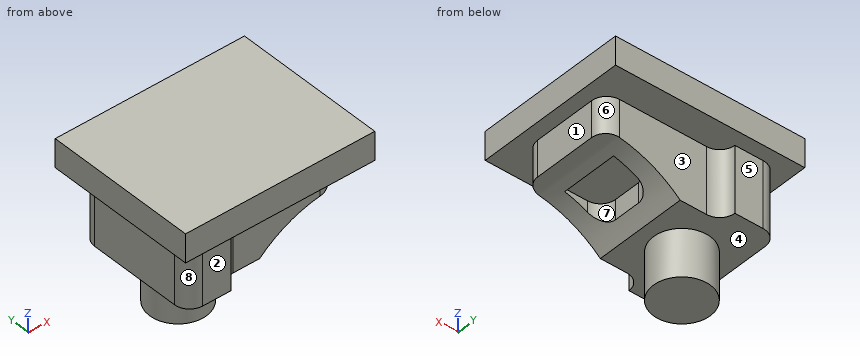
Autodesk Inventor part; units mm, degrees
ref_plane "YZ Plane" through (0, 0, 0) normal (1, 0, 0) x (0, 1, 0)
ref_plane "XZ Plane" through (0, 0, 0) normal (0, 1, 0) x (-1, 0, 0)
ref_plane "XY Plane" through (0, 0, 0) normal (0, 0, 1) x (1, 0, 0)
sketch "Sketch1" plane through (0, 0, 0) normal (0, 0, 1) x (1, 0, 0)
  line L0 (-50, 40) -> (50, 40)
  line L1 (50, 40) -> (50, -40)
  line L2 (50, -40) -> (-50, -40)
  line L3 (-50, -40) -> (-50, 40)
  line L4 (-50, 40) -> (50, -40) construction
  line L5 (50, 40) -> (-50, -40) construction
  line L6 (-34.5, 32.5) -> (-19.5, 32.5)
  line L7 (-19.5, -32.5) -> (-34.5, -32.5)
  line L8 (-42.5, -24.5) -> (-42.5, 24.5)
  line L9 (-42.5, 32.5) -> (-19.5, -32.5) construction
  line L10 (-19.5, 32.5) -> (-42.5, -32.5) construction
  arc A0 (-34.5, 32.5) -> (-42.5, 24.5) centre (-34.5, 24.5) ccw
  arc A1 (-42.5, -24.5) -> (-34.5, -32.5) centre (-34.5, -24.5) ccw
  line L11 (-11.5, 24.5) -> (34.5, 24.5)
  line L12 (42.5, 16.5) -> (42.5, -16.5)
  line L13 (34.5, -24.5) -> (-11.5, -24.5)
  line L14 (-19.5, 24.5) -> (42.5, -24.5) construction
  line L15 (42.5, 24.5) -> (-19.5, -24.5) construction
  arc A2 (42.5, 16.5) -> (34.5, 24.5) centre (34.5, 16.5) ccw
  arc A3 (34.5, -24.5) -> (42.5, -16.5) centre (34.5, -16.5) ccw
  arc A4 (-19.5, 32.5) -> (-11.5, 24.5) centre (-11.5, 32.5) ccw
  arc A5 (-11.5, -24.5) -> (-19.5, -32.5) centre (-11.5, -32.5) ccw
  circle A6 centre (-19.5, 0) radius 15
  line L16 (17.5, 15) -> (29.5, 15)
  line L17 (29.5, 15) -> (29.5, -15)
  line L18 (29.5, -15) -> (17.5, -15)
  line L19 (9.5, -7) -> (9.5, 7)
  line L20 (9.5, 15) -> (29.5, -15) construction
  line L21 (29.5, 15) -> (9.5, -15) construction
  arc A7 (17.5, 15) -> (9.5, 7) centre (17.5, 7) ccw
  arc A8 (9.5, -7) -> (17.5, -15) centre (17.5, -7) ccw
  point P0 (0, 0)
  point P1 (-31, 0)
  point P2 (11.5, 0)
  point P3 (19.5, 0)
  dimension "d0" = 100
  dimension "d1" = 80
  dimension "d2" = 23
  dimension "d3" = 65
  dimension "d4" = 8
  dimension "d5" = 8
  dimension "d6" = 7.5
  dimension "d7" = 62
  dimension "d8" = 49
  dimension "d9" = 7.5
  dimension "d10" = 8
  dimension "d13" = 30
  dimension "d14" = 23
  dimension "d15" = 20
  dimension "d16" = 30
  dimension "d17" = 13
  dimension "d18" = 8
  dimension "d32" = 8
  dimension "d34" = 46
  dimension "d35" = 8
extrude "Extrusion1" add sketch "Sketch1" along normal blind 15 contours L0 L1 L2 L3 | L6 A4 L11 A2 L12 A3 L13 A5 L7 A1 L8 A0 | A6 | L16 L17 L18 A8 L19 A7
extrude "Extrusion2" add sketch "Sketch1" against normal blind 60 contours A6
extrude "Extrusion3" add sketch "Sketch1" against normal blind 35 contours L6 A4 L11 A2 L12 A3 L13 A5 L7 A1 L8 A0
extrude "Extrusion4" add sketch "Sketch1" against normal blind 19 contours L16 L17 L18 A8 L19 A7
sketch "Sketch2" plane through (-11.5, 24.5, 0) normal (0, 1, 0) x (1, 0, 0)
  circle A0 centre (54.7979, 78.9947) radius 60
  line L0 (46, 0) -> (54, 0)
  line L1 (54, 0) -> (54, 19)
  line L2 (54, 0) -> (54, 35)
  line L3 (54, 35) -> (14, 35)
  line L4 (0, 35) -> (46, 35)
  point P0 (11.5, 0)
  dimension "d27" = 120
  dimension "d28" = 19
  dimension "d29" = 40
extrude "Extrusion5" cut sketch "Sketch2" against normal blind 60 contours L3 L2 A0 picked at (26.9594, 33.1676)
properties part number "P2"
Geometry: final body of the model. Coordinates: model frame, mm. Face numbers are marked on the shaded views. A direction names the side the tool comes from. Give positions to 0.01 mm unless a question says otherwise; leave off trailing zeros. Loops run counter-clockwise (first coordinate to the right, second up) from the corner with the lowest first, then second, coordinate; pieces in that order, holes last. Notation, with made-up numbers: (2.25, 70.5) - (11.25, 70.5) arc R13 ccw to (11.25, 82.5) - close; hole circle Ø5 at (87, 23). An arc over 180 degrees is marked (long way). Answer as CSV lines item,"result". Start each with the question number.
1. Section B-B, the plane x = -1. Return loops of the section in (y, z).
2. Ray query, L1, parallel to Z at x = 36.5, y = 25.5; L2, parallel to Z at x = -10, y = -14; L3, parallel to Y at x = -31, z = -1.5. Return the intervals inside material, ascending.
3. Pin query (flat end, axial travel): P1, Ø0.8, axis at y = 3.5, z = -19.5, coming from the -X side; P2, Ø5, axis at y = 18, z = -40.5, coming from the +X side; P3, Ø3, axis at x = 21, z = -21.5, coming from the -Y side; P4, Ø2, axis at x = 13, y = 11, coming from the -Z side. Return the tip coordinate at first contact, or that it passes through.
4. Draft query along Y for the marked faces 6, 7 and 8. Return one class per face: released by +Y, released by -Y, zero draft, split by the parting line, or undercut.
5. Section D-D, the plane y = -22. Return loops of the section in (x, z).
6. Section C-C, the plane y = 0. Return loops of the section in (x, z).
7. Section A-A, the plane z = -15. Return loops of the section in (x, y).
8. Reachability of the marked faces 1, 2, 3, 4 and 5 from +Z, -Z, +X, -X, +Y, -Y: full face, straight path, thin tool, end or side. Return the list, or none.
Answers:
1,outline,"(-40, 0) - (-24.5, 0) - (-24.5, -35) - (24.5, -35) - (24.5, 0) - (40, 0) - (40, 15) - (-40, 15) - close"
2,L1,"z = 0 to 15"
2,L2,"z = -35 to 15"
2,L3,"y = -32.5 to 32.5"
3,P1,"stops at x = -42.5"
3,P2,"passes through"
3,P3,"stops at y = -24.5"
3,P4,"stops at z = -19"
4,face 6,"released by +Y"
4,face 7,"undercut"
4,face 8,"released by -Y"
5,outline,"(-50, 0) - (-42.5, 0) - (-42.5, -35) - (2.5, -35) arc R60 cw to (40.31, -19.07) - (40.31, 0) - (50, 0) - (50, 15) - (-50, 15) - close"
6,outline,"(-50, 0) - (-42.5, 0) - (-42.5, -35) - (-34.5, -35) - (-34.5, -60) - (-4.5, -60) - (-4.5, -35) - (2.5, -35) arc R60 cw to (9.5, -29.42) - (9.5, -19) - (29.5, -19) - (29.5, -20.6) arc R60 cw to (42.5, -19) - (42.5, 0) - (50, 0) - (50, 15) - (-50, 15) - close"
7,outline,"(-42.5, -24.5) arc R8 ccw to (-34.5, -32.5) - (-19.5, -32.5) arc R8 cw to (-11.5, -24.5) - (34.5, -24.5) arc R8 ccw to (42.5, -16.5) - (42.5, 16.5) arc R8 ccw to (34.5, 24.5) - (-11.5, 24.5) arc R8 cw to (-19.5, 32.5) - (-34.5, 32.5) arc R8 ccw to (-42.5, 24.5) - close"
8,face 1,"-Z, +X, +Y, -Y"
8,face 2,"-Z, +X, -X, -Y"
8,face 3,"-Z, +X, +Y"
8,face 4,"-Z"
8,face 5,"-Z, +X, -X, +Y"
